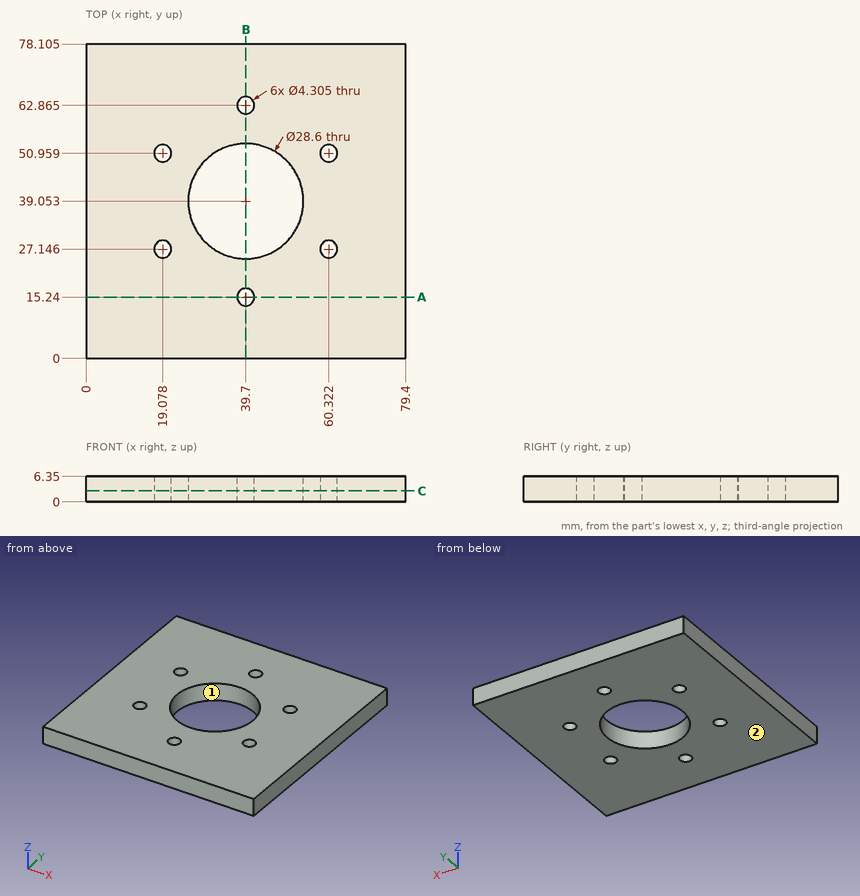
Study the drawing (mm; zero at the part's minimum x, y, z) and answer. Round coordinates to 2 decimals unless told otherwise and drop trailing zeros. Loops run counter-clockwise (first coordinate to the right, second up) from the corner with the lowest first, then second, coordinate; pieces in that order, holes last. Notation, with made-up numbers: (-14.75, 85) -> (43.25, 85) arc R15 cw to (43.25, 96) -> close; hole circle Ø2 at (74, 23). An arc over 180 degrees is marked (long way). Write each question's results on one line, items separated by ' | '. Start each with the question number.
1. Find the intervals of material crossed by probe 1 along Y at (x, z) = (39.7, 1.5) (1 decimal); probe 2 along X at (y, z) = (26, 4.5) (1 decimal); probe 3 along X at (y, z) = (51, 2) (1 decimal), in increasing order. Write a range as from..to.
2. Section B-B (x = 39.7) is taken. State how many separate pieces and enclosed holes the cut face has, plus the area to 3 significant figures.
3. For a pull along Y with two mould halves and no side action, classify the marked faces 1 and 2 as +Y half, -Y half, draft (parallel to the pull), parting line (faces both ways), or undercut.
4. Section A-A (y = 15.24) is taken. Determine the outline of the cut face in (x, z).
5. Section C-C (z = 2.75) is taken. Determine the outline of the cut face in (x, y) (1 decimal), plus the area to 3 significant figures.
Evaluation:
1) probe 1: y = 0..13.1, 17.4..24.8, 53.4..60.7, 65..78.1 | probe 2: x = 0..17.3, 20.9..33.9, 45.5..58.5, 62.1..79.4 | probe 3: x = 0..16.9, 21.2..31.8, 47.6..58.2, 62.5..79.4
2) separate pieces: 4 | enclosed holes: 0 | area: 260 mm2
3) face 1: undercut | face 2: draft
4) outline: (0, 0) -> (37.55, 0) -> (37.55, 6.35) -> (0, 6.35) -> close; (41.85, 0) -> (79.4, 0) -> (79.4, 6.35) -> (41.85, 6.35) -> close
5) outline: (0, 0) -> (79.4, 0) -> (79.4, 78.1) -> (0, 78.1) -> close; hole circle Ø4.3 at (19.1, 27.1); hole circle Ø4.3 at (19.1, 51); hole circle Ø28.6 at (39.7, 39.1); hole circle Ø4.3 at (39.7, 15.2); hole circle Ø4.3 at (39.7, 62.9); hole circle Ø4.3 at (60.3, 27.1); hole circle Ø4.3 at (60.3, 51) | area: 5,470 mm2
